The figure shows three views and two pictorial views of one solid part (mm, origin at its lowest corner). Answer the questions. A direction names the side the tool comes from. Coordinates: 2 decimals unless noted, no trailing zeros. Loops run counter-clockwise (first coordinate to the right, second up) from the corner with the lowest first, then second, coordinate; pieces in that order, holes last. Notation, with made-up numbers: M 44.5,36 L 67.5,36 A21 ccw 67.5,65 Z; hole C -40,-10 d8. An arc over 180 degrees is marked long. One line per item, written item: value. Start each with the question number.
1. Consider probe 1 along Z at (x, y) = (13.25, 1.75); probe 2 along Y at (x, z) = (7, 17.75); probe 3 along Y at (x, z) = (6.5, 15.75). Determine where each line is inside the solid, lowest interval first.
2. For the marked faces 5, 6 and 7, determine the directions among +Z, -Z, +X, -X, +Y, -Y from which every point of the face is accessible in a straight line to the end or side of a thin tool.
3. Determine the mould class of the marked faces 1, 2, 3 and 4 for opening direction Z: +Z half, -Z half, draft (parallel to the pull), parting line (faces both ways), or undercut.
4. The part is cut by section C-C (y = 15.5). Write down the section's boundary in (x, z) (3 decimals).
5. The part is cut by section A-A (y = 12). Write down the section's boundary in (x, z) (3 decimals), then the cut area to 3 significant figures.
6. Flat-ended cylindrical pins translate along their axes: pin 1 (2 mm diameter, centred on x = 10, z = 9, fed in from -Y); pin 2 (2 mm diameter, centred on x = 8, y = 18, fed in from +Z); pin 3 (6 mm diameter, centred on x = 6, z = 17.5, fed in from +Y) (3 decimals); pin 4 (4 mm diameter, centred on y = 14, z = 18, fed in from +X) (3 decimals). Find the tip coordinate at first contact, or state that the pin passes through.
7. The part is cut by section D-D (z = 11). Write down the section's boundary in (x, y), then the cut area to 3 significant figures.
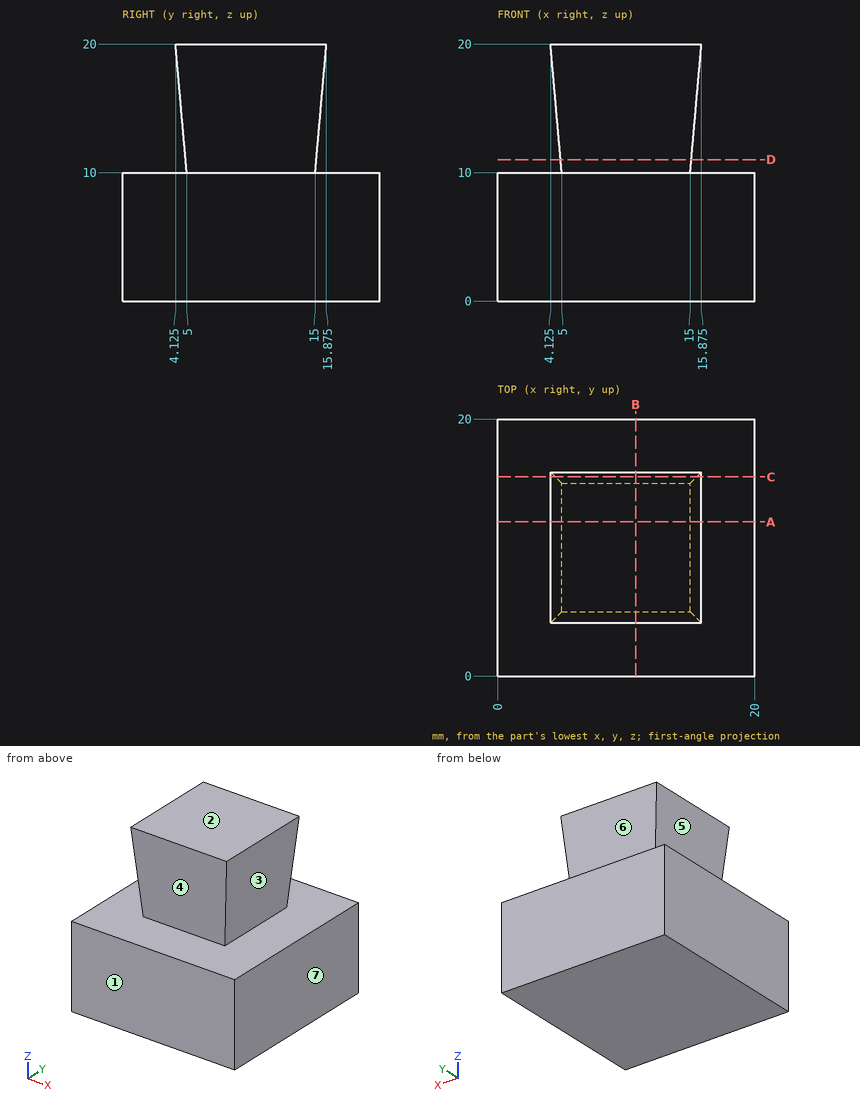
Answer block:
1. probe 1: z = 0 to 10
1. probe 2: y = 4.32 to 15.68
1. probe 3: y = 4.5 to 15.5
2. face 5: -X, +Y, -Y
2. face 6: +X, -X, +Y
2. face 7: +Z, -Z, +X, +Y, -Y
3. face 1: draft
3. face 2: +Z half
3. face 3: undercut
3. face 4: undercut
4. outline: M 0,0 L 20,0 L 20,10 L 0,10 Z; M 4.125,20 L 4.5,15.715 L 15.5,15.715 L 15.875,20 Z
5. outline: M 0,0 L 20,0 L 20,10 L 15,10 L 15.875,20 L 4.125,20 L 5,10 L 0,10 Z
5. area: 309 mm2
6. pin 1: stops at y = 0
6. pin 2: stops at z = 10
6. pin 3: stops at y = 15.875
6. pin 4: stops at x = 15.875
7. outline: M 4.91,4.91 L 15.09,4.91 L 15.09,15.09 L 4.91,15.09 Z
7. area: 104 mm2
